Here's the drawing with two shaded views (mm, measured from the low corner). I have some questions. A direction names the side the tool comes from. Coordinates: 2 decimals unless noted, no trailing zeros. Order: outer loops, then holes, each group sorted by start corner. A loop starts at its lowest first (then second) coordinate and runs counter-clockwise, first axis right, second up. Notation, with made-up numbers: (53, 39) -> (80, 39) arc R27 ccw to (80, 61) -> close; hole circle Ø5 at (-34.75, -35.5). An arc over 180 degrees is marked (long way). Return JSON: item names as keys, results as strings. Group by question number.
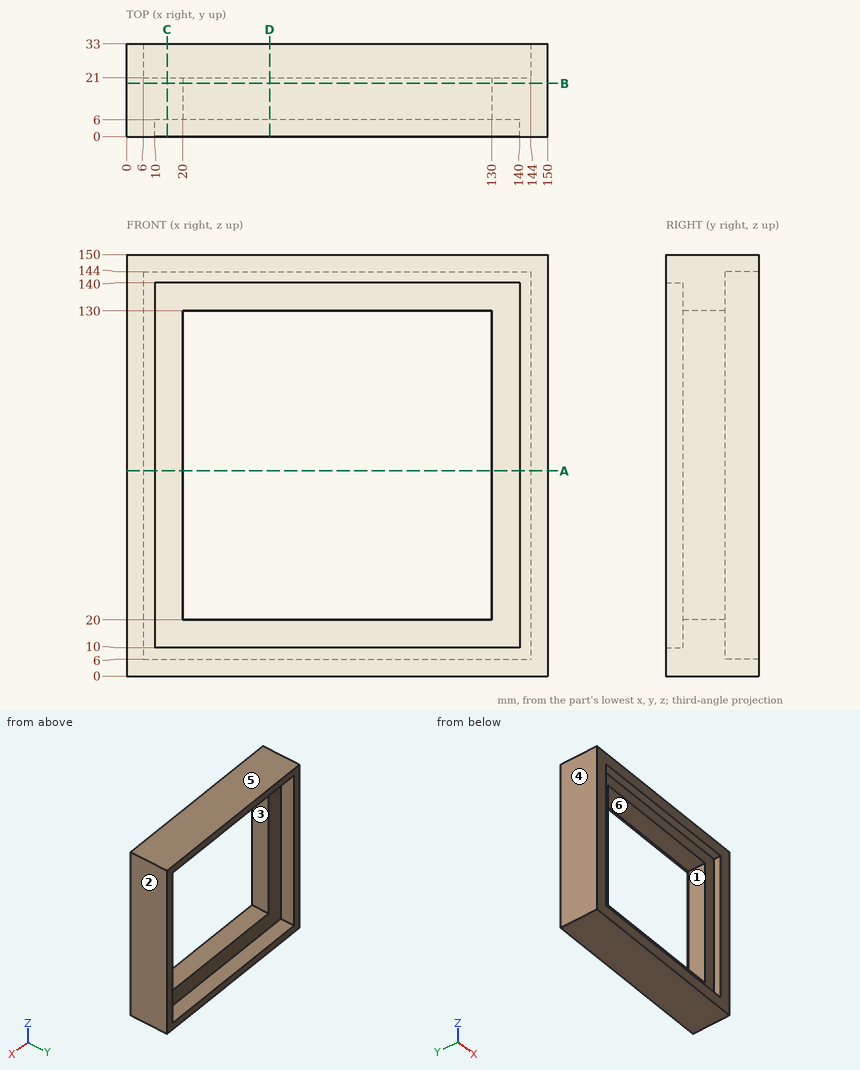
Q1. I want a section at B-B on y = 19. Please give me the cut outline in (x, z), and give its area (3 significant figures).
Q2. I want a section at D-D on x = 51. Please give me the cut outline in (y, z), and give its area (3 significant figures).
Q3. I want a section at C-C on x = 14.5. Please give me the cut outline in (y, z).
Q4. I'm going to push a flat-ended pin straight in: pin 1 Ø12 at (x, z) = (15, 96) entering from +Y. Where does the tip first touch, or does it pass through?
Q5. I want a section at A-A on z = 73. Please give me the cut outline in (x, y).
Q6. On a 3-axis mill with a long thin cutter (end or side, diameter ignored), from which of +Z, -Z, +X, -X, +Y, -Y can I reach the whole of each face in a straight line? I mean the marked faces 1 and 2. Say none if no direction works.
Q7. I need wall thicknesses on line 1 along X through (y, z) = (24.5, 62); line 2 along Z through (x, y) = (77.5, 7). Which ranges of each line are inside material? Lowest first, please. Write a range as from..to.
Q8. We'd pull the mould along Z, two halves only. Please class the marked faces 3, 4, 5 and 6: pulls with the +Z half, pulls with the -Z half, needs draft (parallel to the pull), parting line crosses it, or undercut.
Response values:
{
 "1": {"outline": "(0, 0) -> (150, 0) -> (150, 150) -> (0, 150) -> close; hole (20, 20) -> (130, 20) -> (130, 130) -> (20, 130) -> close", "area": "10,400 mm²"},
 "2": {"outline": "(0, 0) -> (33, 0) -> (33, 6) -> (21, 6) -> (21, 20) -> (6, 20) -> (6, 10) -> (0, 10) -> close; (0, 140) -> (6, 140) -> (6, 130) -> (21, 130) -> (21, 144) -> (33, 144) -> (33, 150) -> (0, 150) -> close", "area": "864 mm²"},
 "3": {"outline": "(0, 0) -> (33, 0) -> (33, 6) -> (21, 6) -> (21, 144) -> (33, 144) -> (33, 150) -> (0, 150) -> (0, 140) -> (6, 140) -> (6, 10) -> (0, 10) -> close"},
 "4": {"pin 1": "stops at y = 21"},
 "5": {"outline": "(0, 0) -> (10, 0) -> (10, 6) -> (20, 6) -> (20, 21) -> (6, 21) -> (6, 33) -> (0, 33) -> close; (130, 6) -> (140, 6) -> (140, 0) -> (150, 0) -> (150, 33) -> (144, 33) -> (144, 21) -> (130, 21) -> close"},
 "6": {"face 1": "+Y, -Y", "face 2": "+Z, -Z, +X, +Y, -Y"},
 "7": {"line 1": "x = 0..6, 144..150", "line 2": "z = 0..20, 130..150"},
 "8": {"face 3": "undercut", "face 4": "needs draft", "face 5": "pulls with the +Z half", "face 6": "undercut"}
}
